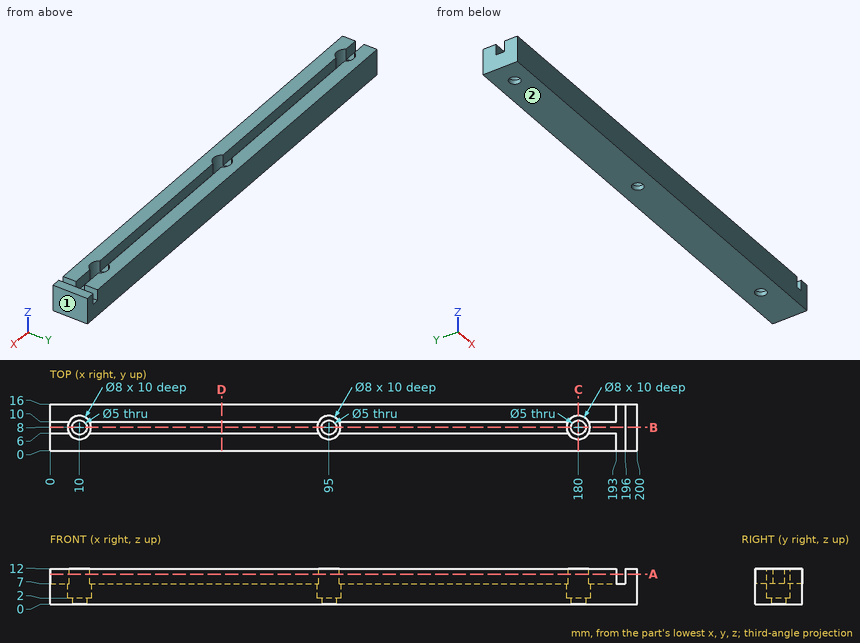
Geometry check sheet. Reference: drawing and pictorial views, mm from the part's lowest x, y, z. Coordinates: 2 decimals unless noted, no trailing zeros. Write each loop counter-clockwise with the first axis right and the second up, starting at its lowest first coordinate (ties: lowest second). Pieces come first, ordered by that corner, then holes. Notation, with made-up numbers: M 63.25,-30 L 71.25,-30 A23 cw 71.25,-7 Z; hole C 41.25,-21.75 d4. An arc over 180 degrees is marked long. One line per question, with ' | ' between items.
1) Depth check by flat-ended pin: pin 1 Ø1.2 at (x, y) = (133, 8.5) entering from +Z; pin 2 Ø1.5 at (y, z) = (9.5, 4) entering from -X; pin 3 Ø6 at (x, y) = (180, 8) entering from +Z. Enter the tip coordinate at first touch or a pass-through.
Solutions:
pin 1: z = 7 | pin 2: x = 0 | pin 3: z = 2
2) Sectioned sample at D-D on x = 58.5. Record the cut outline in (y, z).
Solutions:
outline: M 0,0 L 16,0 L 16,12 L 10,12 L 10,7 L 6,7 L 6,12 L 0,12 Z
3) Sectioned sample at A-A on z = 10.25. Record the cut outline in (x, y).
Solutions:
outline: M 0,0 L 193,0 L 193,6 L 183.46,6 A4 cw 176.54,6 L 98.46,6 A4 cw 91.54,6 L 13.46,6 A4 cw 6.54,6 L 0,6 Z; M 0,10 L 6.54,10 A4 cw 13.46,10 L 91.54,10 A4 cw 98.46,10 L 176.54,10 A4 cw 183.46,10 L 193,10 L 193,16 L 0,16 Z; M 196,0 L 200,0 L 200,16 L 196,16 Z
4) Sectioned sample at C-C on x = 180. Record the cut outline in (y, z), then the cut area to 3 significant figures.
Solutions:
outline: M 0,0 L 5.5,0 L 5.5,2 L 4,2 L 4,12 L 0,12 Z; M 10.5,0 L 16,0 L 16,12 L 12,12 L 12,2 L 10.5,2 Z | area: 102 mm^2
5) Sectioned sample at B-B on y = 8. State how many separate pieces and enclosed holes the cut face has, then the cut area to 3 significant figures.
Solutions:
separate pieces: 4 | enclosed holes: 0 | area: 1,270 mm^2
6) Release check for a two-part mould opening along Z. For the marked faces 1 and 2 record: +Z half, -Z half, draft (parallel to the pull), parting line (faces both ways), or undercut.
Solutions:
face 1: draft | face 2: -Z half
7) Material ranges on L1, parallel to X at y = 8, z = 6.75; L2, parallel to Y at x = 95, z = 7.75; L3, parallel to Y at x = 10, z = 1.1, recorded low to high.
Solutions:
L1: 0 to 6, 14 to 91, 99 to 176, 184 to 200 | L2: 0 to 4, 12 to 16 | L3: 0 to 5.5, 10.5 to 16
